Design review of the part built by this model. Coordinates are the model's own, in mm. A direction names the side the tool comes from. Coordinates: 2 decimals unless noted, no trailing zeros. Order: outer loops, then holes, each group sorted by start corner. A loop starts at its lowest first (then second) coordinate and runs counter-clockwise, first axis right, second up. Notation, with made-up numbers: M 2,44.25 L 47,44.25 A26 ccw 47,74.25 Z; hole C -2,49 d3. An arc over 180 degrees is marked long. Answer as a JSON object with one key per item and string values.
from build123d import *

# Parameters (mm, degrees)
SKETCH057_W         = 21.5
SKETCH057_H         = 41.5
PAD033_DEPTH        = 6
SKETCH056_W         = 17.5
SKETCH056_H         = 37.5
POCKET018_DEPTH     = 4
SKETCH059_W         = 13.5
SKETCH059_H         = 33.5
POCKET019_DEPTH     = 2.001
SKETCH058_W         = 11.5
SKETCH058_H         = 4
POCKET017_DEPTH     = 6.001
REVOLUTION003_ANGLE = 180
REVOLUTION004_ANGLE = 180


with BuildPart() as part:
    # Sketch057 → Pad033 (new body)
    with BuildSketch(Plane.XY):
        with Locations((10.75, 20.75)):
            Rectangle(SKETCH057_W, SKETCH057_H)
    extrude(amount=PAD033_DEPTH)

    # Sketch056 (on Face6 of Pad033) → Pocket018 (cut)
    with BuildSketch(Plane.XY.offset(6)):
        with Locations((10.75, 20.75)):
            Rectangle(SKETCH056_W, SKETCH056_H)
    extrude(amount=-POCKET018_DEPTH, mode=Mode.SUBTRACT)

    # Sketch059 (on Face11 of Pocket018) → Pocket019 (cut, through all)
    with BuildSketch(Plane.XY.offset(2)):
        with Locations((10.75, 20.75)):
            Rectangle(SKETCH059_W, SKETCH059_H)
    extrude(amount=-POCKET019_DEPTH, mode=Mode.SUBTRACT)

    # Sketch058 (on Face5 of Pocket019) → Pocket017 (cut, through all)
    with BuildSketch(Plane.XY.offset(6)):
        with Locations((10.75, 2)):
            Rectangle(SKETCH058_W, SKETCH058_H)
    extrude(amount=-POCKET017_DEPTH, mode=Mode.SUBTRACT)

    # Sketch060 (on Face20 of Pocket017) → Revolution003 (revolve)
    with BuildSketch(Plane.YZ.offset(2)):
        with BuildLine():
            ThreePointArc((5, 5), (4, 6), (3, 5))
            Line((3, 5), (5, 5))
        make_face()
        with BuildLine():
            ThreePointArc((38.5, 5), (37.5, 6), (36.5, 5))
            Line((36.5, 5), (38.5, 5))
        make_face()
    revolve(axis=Axis((2, 5, 5), (0, 1, 0)), revolution_arc=REVOLUTION003_ANGLE)

    # Sketch061 (on Face19 of Revolution003) → Revolution004 (revolve)
    with BuildSketch(Plane(origin=(19.5, 0, 0), x_dir=(0, -1, 0), z_dir=(-1, 0, 0))):
        with BuildLine():
            ThreePointArc((-36.5, 5), (-37.5, 6), (-38.5, 5))
            Line((-38.5, 5), (-36.5, 5))
        make_face()
        with BuildLine():
            ThreePointArc((-3, 5), (-4, 6), (-5, 5))
            Line((-5, 5), (-3, 5))
        make_face()
    revolve(axis=Axis((19.5, 36.5, 5), (0, -1, 0)), revolution_arc=REVOLUTION004_ANGLE)


solid = part.part
1) Tool access review of faces 4 (the flat face through (0, 20, 3)), 5 (the flat face through (5, 1.5, 2.4)), 6 (the flat face through (11, 37.5, 1)): name each direction out of +Z, -Z, +X, -X, +Y, -Y from which nothing blocks a thin tool from reaching the whole face with its end or side.
Taken from the geometry:
{"face 4": "+Z, -Z, -X, +Y, -Y", "face 5": "+Z, -Z, -Y", "face 6": "+Z, -Z"}
2) Insertion check: pin 1 Ø0.6 at (x, z) = (8, 1) entering from -Y; pin 2 Ø2 at (x, z) = (6.5, 3.5) entering from -Y. Each pin has a flat end and moves straight along its axis. Give the tip position at first contact, or say it passes through.
Taken from the geometry:
{"pin 1": "stops at y = 37.5", "pin 2": "stops at y = 39.5"}
3) Add section C-C (x = 3.5). State the section outline as (y, z) points, and give its area (3 significant figures).
Taken from the geometry:
{"outline": "M 0,0 L 41.5,0 L 41.5,6 L 39.5,6 L 39.5,2 L 2,2 L 2,6 L 0,6 Z", "area": "99.0 mm2"}
4) Add section D-D (z = 2.8). State the section outline as (x, y) points.
Taken from the geometry:
{"outline": "M 0,0 L 5,0 L 5,2 L 2,2 L 2,39.5 L 19.5,39.5 L 19.5,2 L 16.5,2 L 16.5,0 L 21.5,0 L 21.5,41.5 L 0,41.5 Z"}
5) Add section A-A (y = 32). State the section outline as (x, z) points, and give its area (3 significant figures).
Taken from the geometry:
{"outline": "M 0,0 L 4,0 L 4,2 L 2,2 L 2,6 L 0,6 Z; M 17.5,0 L 21.5,0 L 21.5,6 L 19.5,6 L 19.5,2 L 17.5,2 Z", "area": "32.0 mm2"}
6) Add section B-B (z = 0.75). State the section outline as (x, y) points, and give its area (3 significant figures).
Taken from the geometry:
{"outline": "M 0,0 L 5,0 L 5,4 L 4,4 L 4,37.5 L 17.5,37.5 L 17.5,4 L 16.5,4 L 16.5,0 L 21.5,0 L 21.5,41.5 L 0,41.5 Z", "area": "394 mm2"}
7) To check wall thickness, follow L1, parallel to Y at x = 4.5, z = 0.4; L2, parallel to X at y = 26.5, z = 3.75; L3, parallel to Y at x = 17.75, z = 4.75. State the ranges of each line that lie inside material, in increasing order.
Taken from the geometry:
{"L1": "y = 0 to 4, 37.5 to 41.5", "L2": "x = 0 to 2, 19.5 to 21.5", "L3": "y = 0 to 2, 39.5 to 41.5"}
8) Mouldability with a two-part tool opening along Y and no side actions: class faces 1 (the flat face through (16.5, 1.5, 2.4)), 2 (the flat face through (19, 0, 3)), 3 (the flat face through (2, 20, 4)) as released by +Y, released by -Y, zero draft, split by the parting line, or undercut.
Taken from the geometry:
{"face 1": "zero draft", "face 2": "released by -Y", "face 3": "undercut"}
